Design review of the part built by this model. Coordinates are the model's own, in mm. Face numbers are marked on the shaded views. A direction names the side the tool comes from. Give positions to 0.01 mm unless a question says otherwise; leave off trailing zeros. Loops run counter-clockwise (first coordinate to the right, second up) from the corner with the lowest first, then second, coordinate; pieces in that order, holes last. Notation, with made-up numbers: (11.5, 51) - (52.5, 51) arc R27 ccw to (52.5, 77) - close; hole circle Ø11 at (19, 87.5). An arc over 180 degrees is marked (long way). Write each question's results on one line, items separated by ' | '.
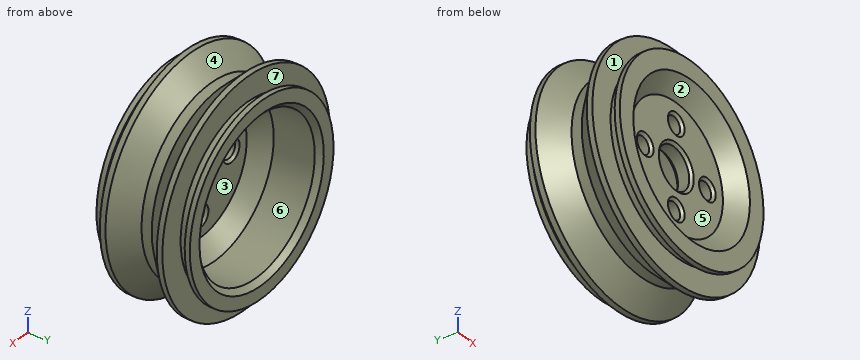
from build123d import *

# Parameters (mm, degrees)
SKETCH_1_R               = 21.6
EXTRUDE_1_DEPTH          = 9.1
SKETCH_2_W               = 4.7
SKETCH_2_H               = 2
SKETCH_2_W_2             = 3.1
SKETCH_2_H_2             = 1
SKETCH_3_R               = 15
CUT_EXTRUDE_1_DEPTH      = 3
SKETCH_4_R               = 4
CUT_EXTRUDE_2_DEPTH      = 20
SKETCH_5_R               = 1.65
CUT_EXTRUDE_3_DEPTH      = 20
PATTERN_CIRCULAR_1_COUNT = 4
CUT_EXTRUDE_START        = -6.2
SKETCH_3_2_R             = 15
CUT_EXTRUDE_4_DEPTH      = 12
SKETCH_6_W               = 4
SKETCH_6_H               = 10
CHAMFER_1_SIZE           = 4
CHAMFER_2_SIZE           = 3
CHAMFER_3_SIZE           = 1
CHAMFER_4_SIZE           = 0.5


with BuildPart() as part:
    # 草图1 → 凸台-拉伸1 (new, symmetric)
    with BuildSketch(Plane(origin=(0, 0, 0), x_dir=(1, 0, 0), z_dir=(0, 1, 0))):
        with Locations(Location((0, 0, 0), (0, 0, 270))):
            Circle(SKETCH_1_R)
    extrude(amount=EXTRUDE_1_DEPTH, both=True)

    # 草图2 → 切除-旋转1 (revolve, cut)
    with BuildSketch(Plane.XY, mode=Mode.PRIVATE) as cut_revolve_1_sk:
        with Locations((19.25, -7.1)):
            Rectangle(SKETCH_2_W, SKETCH_2_H)
        with Locations((20.05, -8.6)):
            Rectangle(SKETCH_2_W_2, SKETCH_2_H_2)
    cut_revolve_1 = revolve(cut_revolve_1_sk.sketch.rotate(Axis((0, 9.1, 0), (0, -1, 0)), 90), axis=Axis((0, 9.1, 0), (0, -1, 0)), mode=Mode.SUBTRACT)

    # 镜向1: 切除-旋转1 across plane
    add(cut_revolve_1.mirror(Plane.ZX), mode=Mode.SUBTRACT)

    # 草图3 → 切除-拉伸1 (cut)
    with BuildSketch(Plane.XZ.offset(9.1)):
        with Locations(Location((0, 0, 0), (0, 0, 270))):
            Circle(SKETCH_3_R)
    extrude(amount=-CUT_EXTRUDE_1_DEPTH, mode=Mode.SUBTRACT)

    # 草图4 → 切除-拉伸2 (cut)
    with BuildSketch(Plane.XZ.offset(6.1)):
        with Locations(Location((0, 0, 0), (0, 0, 270))):
            Circle(SKETCH_4_R)
    extrude(amount=-CUT_EXTRUDE_2_DEPTH, mode=Mode.SUBTRACT)

    # 草图5 → 切除-拉伸3 (cut)
    with BuildSketch(Plane.XZ.offset(6.1)):
        with Locations(Location((-8, 0, 0), (0, 0, 270))):
            Circle(SKETCH_5_R)
    cut_extrude_3 = extrude(amount=-CUT_EXTRUDE_3_DEPTH, mode=Mode.SUBTRACT)

    # 阵列(圆周)1: 切除-拉伸3 ×4 about axis
    pattern_circular_1_axis = Axis((0, 0, 0), (0, 1, 0))
    for i in range(1, PATTERN_CIRCULAR_1_COUNT):
        add(cut_extrude_3.rotate(pattern_circular_1_axis, i * 360 / PATTERN_CIRCULAR_1_COUNT), mode=Mode.SUBTRACT)

    # 草图3<2> → 切除-拉伸4 (cut)
    with BuildSketch(Plane.XZ.offset(9.1).offset(CUT_EXTRUDE_START)):
        with Locations(Location((0, 0, 0), (0, 0, 270))):
            Circle(SKETCH_3_2_R)
    extrude(amount=-CUT_EXTRUDE_4_DEPTH, mode=Mode.SUBTRACT)

    # 草图6 → 切除-旋转2 (revolve, cut)
    with BuildSketch(Plane.XY, mode=Mode.PRIVATE) as cut_revolve_2_sk:
        with Locations((19.6, 0)):
            Rectangle(SKETCH_6_W, SKETCH_6_H)
    revolve(cut_revolve_2_sk.sketch.rotate(Axis((0, 9.1, 0), (0, -1, 0)), 90), axis=Axis((0, 9.1, 0), (0, -1, 0)), mode=Mode.SUBTRACT)

    # 倒角1
    chamfer_1_edges = [part.edges().sort_by_distance(p)[0] for p in [
        (0, -5, -17.6),
        (0, 5, -17.6),
    ]]
    chamfer(chamfer_1_edges, length=CHAMFER_1_SIZE - 0.0001)  # a hair under: the kernel refuses the full size

    # 倒角2
    chamfer_2_edges = [part.edges().sort_by_distance(p)[0] for p in [
        (0, -6.1, 15),
        (0, -2.9, 15),
    ]]
    chamfer(chamfer_2_edges, length=CHAMFER_2_SIZE - 0.0001)  # a hair under: the kernel refuses the full size

    # 倒角3
    chamfer_3_edges = [part.edges().sort_by_distance(p)[0] for p in [
        (0, 9.1, 15),
    ]]
    chamfer(chamfer_3_edges, length=CHAMFER_3_SIZE)

    # 倒角4
    chamfer_4_edges = [part.edges().sort_by_distance(p)[0] for p in [
        (0, -6.1, 4),
        (-8, -6.1, 1.65),
        (-1.65, -6.1, -8),
        (8, -6.1, -1.65),
        (1.65, -6.1, 8),
        (0, -2.9, 4),
        (-8, -2.9, 1.65),
        (1.65, -2.9, 8),
        (8, -2.9, -1.65),
        (-1.65, -2.9, -8),
    ]]
    chamfer(chamfer_4_edges, length=CHAMFER_4_SIZE)


solid = part.part
(1) Take a section at A-A on x = 0. Count the separate pieces of the cut face and the enclosed holes in it, plus the area to 3 significant figures.
Answers below:
separate pieces: 4 | enclosed holes: 0 | area: 207 mm2
(2) Tool access review of the marked faces 5, 6 and 7: name each direction out of +Z, -Z, +X, -X, +Y, -Y from which nothing blocks a thin tool from reaching the whole face with its end or side.
Answers below:
face 5: -Y | face 6: +Y | face 7: none
(3) Insertion check: P1, Ø1.5, axis at x = 16.5, y = 3, coming from the +Z side; P2, Ø10.5, axis at x = 0, z = 0, coming from the +Y side; P3, Ø1.5, axis at y = 3.5, z = 15.5, coming from the +X side; P4, Ø3, axis at x = 0, z = -8, coming from the -Y side. Each pin has a flat end and moves straight along its axis. Give the tip position at first contact, or say it passes through.
Answers below:
P1: z = 12.27 | P2: y = -2.9 | P3: x = 14.21 | P4: through
(4) Wall thickness on line 1 along Y through (x, z) = (2, 18); line 2 along X through (y, z) = (-4.7, 0); line 3 along Y through (x, z) = (9.5, -4): over which ranges is each line inside the solid? List them lowest first. Write a range as from..to.
Answers below:
line 1: -9.1..-8.1, -6.1..-1.51, 1.51..6.1, 8.1..9.1 | line 2: -21.3..-9.65, -6.35..-4, 4..6.35, 9.65..21.3 | line 3: -6.1..-2.9
(5) Take a section at B-B on y = 2.5. Give the boundary of the cut face in (x, z).
Answers below:
outline: circle Ø38.2 at (0, 0); hole circle Ø30 at (0, 0)
(6) Draft analysis for pull direction Z (two halves, no side actions). For the marked faces 1, 2, 3 and 4, state which applies: pulls with the +Z half, pulls with the -Z half, needs draft (parallel to the pull), parting line crosses it, or undercut.
Answers below:
face 1: needs draft | face 2: undercut | face 3: undercut | face 4: parting line crosses it
(7) Take a section at D-D on y = -1.75. Give the boundary of the cut face in (x, z).
Answers below:
outline: circle Ø36.7 at (0, 0); hole circle Ø26.3 at (0, 0)
